Geometry: see drawing. Coordinates: mm, zero at the bounding-box minimum. A direction names the side the tool comes from. Coordinates: 2 decimals unless noted, no trailing zeros. Write each loop counter-clockwise with the first axis right and the second up, starting at its lowest first coordinate (ties: lowest second). Pieces come first, ordered by that corner, then holes. Notation, with made-up numbers: M -2.5,46 L 37.5,46 A19 ccw 37.5,72 Z; hole C 27,33.25 d4. An arc over 180 degrees is marked long. One line per item, written item: value. Start each with the question number.
Item 1: Cut plane A-A, the plane x = 6.7. Output: boundary loops of the cut face in (y, z), then the cut area to 3 significant figures.
Item 2: Ray query, L1, parallel to Y at x = 2.5, z = 10; L2, parallel to Y at x = 6.75, z = 9; L3, parallel to Z at x = 6.75, y = 8. Return the intervals inside material, ascending. Write a range as from..to.
Item 3: Set-up query: the marked faces 1, 2 and 3. Return all of +Z, -Z, +X, -X, +Y, -Y with unobstructed straight access to the full face (end or side cutting, diameter ignored); none if empty.
Item 4: Cut plane C-C, the plane x = 4.75. Output: boundary loops of the cut face in (y, z).
Item 5: Cut plane B-B, the plane z = 6.5. Output: boundary loops of the cut face in (x, y).
Item 6: Cut plane D-D, the plane z = 4. Output: boundary loops of the cut face in (x, y).
Item 7: Pin query (flat end, axial travel): P1, Ø6, axis at x = 10.5, y = 16.5, coming from the -Z side; P2, Ø1.7, axis at x = 6.5, z = 9, coming from the +Y side; P3, Ø5, axis at x = 5.5, y = 18.5, coming from the +Z side. Return the tip coordinate at first contact, or that it passes through.
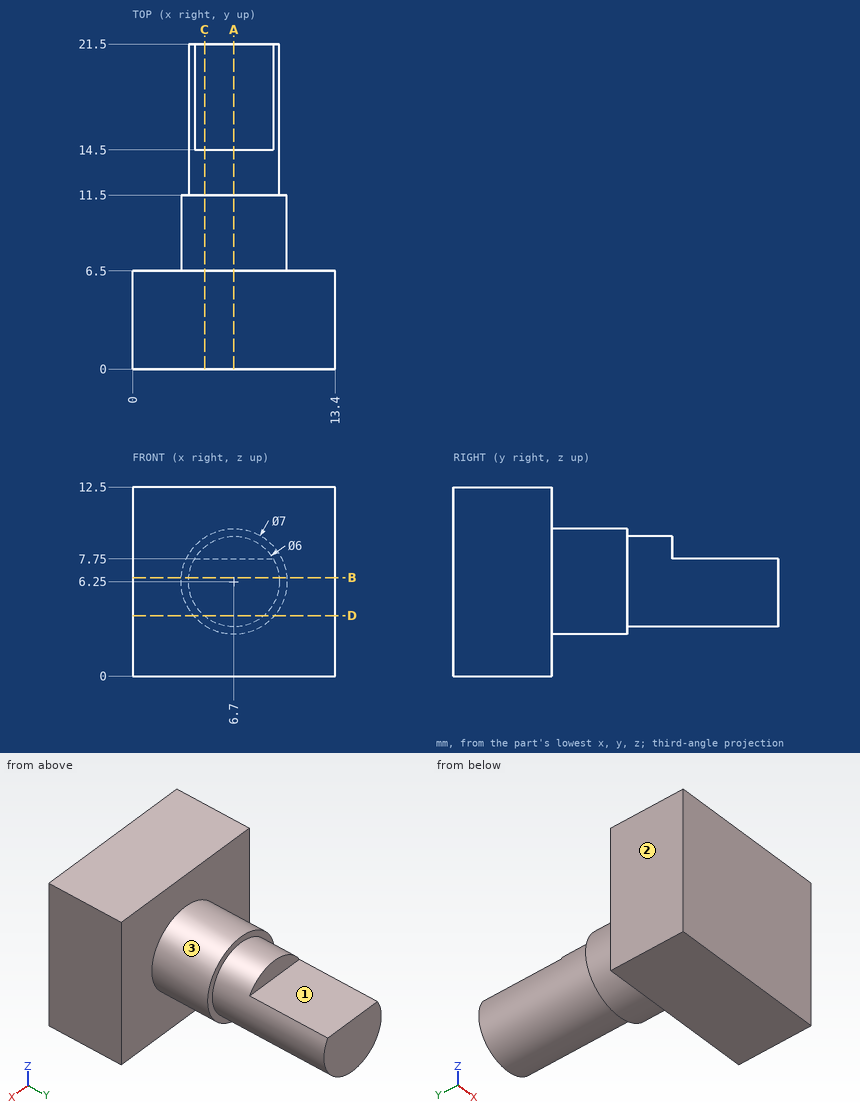
From the geometry:
1. outline: M 0,0 L 6.5,0 L 6.5,2.75 L 11.5,2.75 L 11.5,3.25 L 21.5,3.25 L 21.5,7.75 L 14.5,7.75 L 14.5,9.25 L 11.5,9.25 L 11.5,9.75 L 6.5,9.75 L 6.5,12.5 L 0,12.5 Z
1. area: 166 mm²
2. L1: y = 0..6.5
2. L2: y = 0..14.5
2. L3: z = 2.75..9.75
3. face 1: +Z, +X, -X, +Y
3. face 2: +Z, -Z, -X, +Y, -Y
3. face 3: +Y
4. outline: M 0,0 L 6.5,0 L 6.5,3.34 L 11.5,3.34 L 11.5,3.97 L 21.5,3.97 L 21.5,7.75 L 14.5,7.75 L 14.5,8.53 L 11.5,8.53 L 11.5,9.16 L 6.5,9.16 L 6.5,12.5 L 0,12.5 Z
5. outline: M 0,0 L 13.4,0 L 13.4,6.5 L 10.19,6.5 L 10.19,11.5 L 9.69,11.5 L 9.69,21.5 L 3.71,21.5 L 3.71,11.5 L 3.21,11.5 L 3.21,6.5 L 0,6.5 Z
6. outline: M 0,0 L 13.4,0 L 13.4,6.5 L 9.38,6.5 L 9.38,11.5 L 8.68,11.5 L 8.68,21.5 L 4.72,21.5 L 4.72,11.5 L 4.02,11.5 L 4.02,6.5 L 0,6.5 Z
7. P1: stops at z = 3.36
7. P2: stops at y = 14.5
7. P3: stops at z = 7.75
